from build123d import *

# Parameters (mm, degrees)
SKETCH1_W           = 350
SKETCH1_H           = 150
BOSS_EXTRUDE1_DEPTH = 10
FILLET2_R           = 10
SKETCH9_W           = 120.821087965
SKETCH9_H           = 9.816766212
CUT_EXTRUDE6_DEPTH  = 25


with BuildPart() as part:
    # Sketch1 → Boss-Extrude1 (new body)
    with BuildSketch(Plane(origin=(0, 0, 0), x_dir=(1, 0, 0), z_dir=(0, 1, 0))):
        with Locations((175, -75)):
            Rectangle(SKETCH1_W, SKETCH1_H)
    extrude(amount=BOSS_EXTRUDE1_DEPTH)

    # Fillet2
    fillet2_edges = [part.edges().sort_by_distance(p)[0] for p in [
        (0, 5, 0),
        (350, 5, 0),
        (350, 5, 150),
        (0, 5, 150),
    ]]
    fillet(fillet2_edges, radius=FILLET2_R)

    # Sketch9 → Cut-Extrude6 (cut)
    with BuildSketch(Plane(origin=(0, 10, 0), x_dir=(1, 0, 0), z_dir=(0, 1, 0))):
        with Locations((244.170878002, -145.091616894)):
            Rectangle(SKETCH9_W, SKETCH9_H)
        with Locations((244.170878002, -4.908383106)):
            Rectangle(SKETCH9_W, SKETCH9_H)
    extrude(amount=-CUT_EXTRUDE6_DEPTH, mode=Mode.SUBTRACT)


solid = part.part
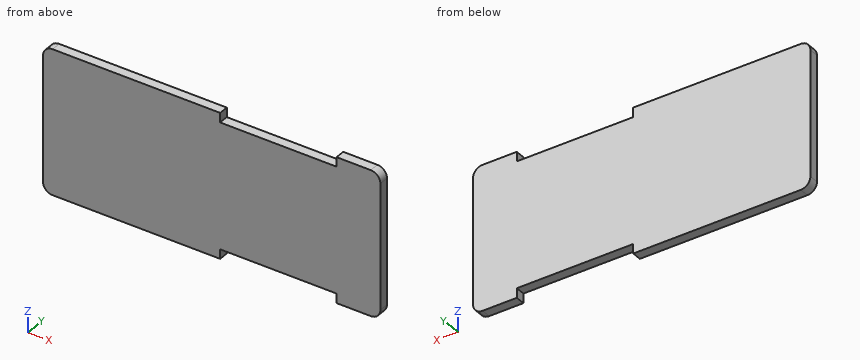
Verification items for the finished model (mm, model axes). Coordinates: 2 decimals unless noted, no trailing zeros. Order: outer loops, then holes, each group sorted by start corner. A loop starts at its lowest first (then second) coordinate and runs counter-clockwise, first axis right, second up. Notation, with made-up numbers: M 35.5,-37 L 57.5,-37 A23 cw 57.5,-4 Z; hole C 22.5,-0.75 d4. An arc over 180 degrees is marked long. One line per item, written item: value. Start each with the question number.
Item 1: Sectioned sample at B-B (x = 200). Enter the section's corners in (y, z), then the cut area to 3 significant figures.
Item 2: Sectioned sample at A-A (y = 4). Enter the section's corners in (x, z).
Item 3: Scan line: probe 1 along Z at (x, y) = (218, 1.75). Record every from-to range of solid material in increasing order.
Item 4: Gauge pin test, flat ends, axial feed: pin 1 (5 mm diameter, centred on y = 6, z = 4.5, fed in from -X); pin 2 (6 mm diameter, centred on x = 212.5, z = 121.5, fed in from -Y); pin 3 (2 mm diameter, centred on x = 265.5, y = 7.5, fed in from -Z); pin 4 (5 mm diameter, centred on y = 7, z = 145, fed in from -X). Record the tip position at first contact, or that the pin passes through.
Conclusion:
1. outline: M 0,9.82 L 10,9.82 L 10,140.18 L 0,140.18 Z
1. area: 1,300 mm^2
2. outline: M 0,10 A10 ccw 10,0 L 183.76,0 L 183.76,9.82 L 304.58,9.82 L 304.58,0 L 340,0 A10 ccw 350,10 L 350,140 A10 ccw 340,150 L 304.58,150 L 304.58,140.18 L 183.76,140.18 L 183.76,150 L 10,150 A10 ccw 0,140 Z
3. probe 1: z = 9.82 to 140.18
4. pin 1: stops at x = 0.46
4. pin 2: stops at y = 0
4. pin 3: stops at z = 9.82
4. pin 4: stops at x = 0.32
